```python
from build123d import *

# Parameters (mm, degrees)
SKETCH_R     = 1
PAD_DEPTH    = 0.4
SKETCH001_R  = 0.75
PAD001_DEPTH = 4.6
SKETCH002_R  = 0.45
PAD002_DEPTH = 2
SKETCH003_R  = 0.3
PAD003_DEPTH = 1.4
CHAMFER_SIZE = 0.05
FILLET_R     = 0.1
FILLET001_R  = 0.45


with BuildPart() as part:
    # Sketch → Pad (new body)
    with BuildSketch(Plane.XY):
        Circle(SKETCH_R)
    extrude(amount=PAD_DEPTH)

    # Sketch001 (on Face3 of Pad) → Pad001 (join)
    with BuildSketch(Plane.XY.offset(0.4)):
        Circle(SKETCH001_R)
    extrude(amount=PAD001_DEPTH)

    # Sketch002 (on Face5 of Pad001) → Pad002 (join)
    with BuildSketch(Plane.XY.offset(5)):
        Circle(SKETCH002_R)
    extrude(amount=PAD002_DEPTH)

    # Sketch003 (on Face2 of Pad002) → Pad003 (join)
    with BuildSketch(Plane(origin=(0, 0, 0), x_dir=(1, 0, 0), z_dir=(0, 0, -1))):
        Circle(SKETCH003_R)
    extrude(amount=PAD003_DEPTH)

    # Chamfer
    chamfer_edges = [part.edges().sort_by_distance(p)[0] for p in [
        (-1, 0, 0),
    ]]
    chamfer(chamfer_edges, length=CHAMFER_SIZE)

    # Fillet
    fillet_edges = [part.edges().sort_by_distance(p)[0] for p in [
        (-0.75, 0, 5),
    ]]
    fillet(fillet_edges, radius=FILLET_R)

    # Fillet001
    fillet001_edges = [part.edges().sort_by_distance(p)[0] for p in [
        (-0.45, 0, 7),
    ]]
    fillet(fillet001_edges, radius=FILLET001_R)


solid = part.part
```
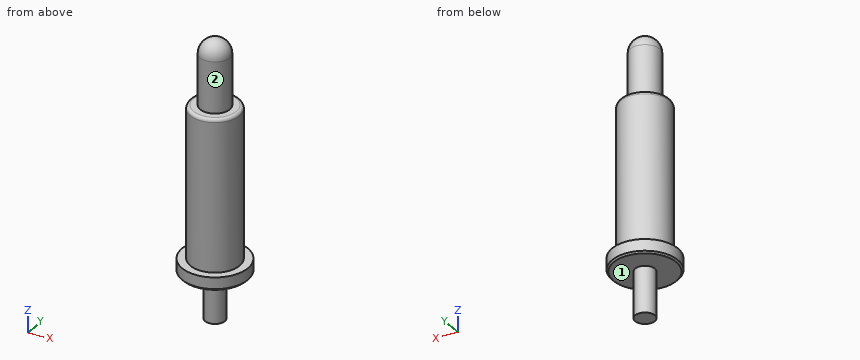
Model file for the job. Use its own axes, mm. Face numbers are marked on the shaded views. A direction names the side the tool comes from. Give positions to 0.01 mm unless a question says otherwise; leave off trailing zeros. Order: outer loops, then holes, each group sorted by start corner. A loop starts at its lowest first (then second) coordinate and runs counter-clockwise, first axis right, second up.
1) Saw through at A-A, the plane y = 0. Write the cut outline in (x, z).
2) Pin check, flat tip, straight feed: pin 1 (1 mm diameter, centred on x = -1, y = -0.5, fed in from +Z). Stop position of the tip, or through.
3) Saw through at C-C, the plane z = 4.5. Write the cut outline in (x, y), then the cut area to 3 significant figures.
4) Wall check: probe 1 along Y at (x, z) = (0.6, 3.5); probe 2 along Z at (x, y) = (-0.5, -0.45); probe 3 along Y at (x, z) = (0, 1.5). Give the ranges that are in metal, low to high.
5) 3-axis set-ups, long thin cutter, end or side, ignore diameter. For the marked faces 1 and 2: which of +Z, -Z, +X, -X, +Y, -Y reach the whole face in a straight line?
Computed:
1. outline: (-1, 0.05) - (-0.95, 0) - (-0.3, 0) - (-0.3, -1.4) - (0.3, -1.4) - (0.3, 0) - (0.95, 0) - (1, 0.05) - (1, 0.4) - (0.75, 0.4) - (0.75, 4.9) arc R0.1 ccw to (0.65, 5) - (0.45, 5) - (0.45, 6.55) arc R0.45 ccw to (-0.45, 6.55) - (-0.45, 5) - (-0.65, 5) arc R0.1 ccw to (-0.75, 4.9) - (-0.75, 0.4) - (-1, 0.4) - close
2. pin 1: stops at z = 5
3. outline: circle Ø1.5 at (0, 0)
3. area: 1.77 mm2
4. probe 1: y = -0.45 to 0.45
4. probe 2: z = 0 to 5
4. probe 3: y = -0.75 to 0.75
5. face 1: -Z
5. face 2: +Z
